Design review of the part built by this model. Coordinates are the model's own, in mm. A direction names the side the tool comes from. Give positions to 0.01 mm unless a question says otherwise; leave off trailing zeros. Write each loop counter-clockwise with the first axis right and the second up, starting at its lowest first coordinate (ties: lowest second). Pieces come first, ordered by that corner, then holes. Notation, with made-up numbers: (-23, -32.5) - (-7, -32.5) arc R10 ccw to (-7, -16.5) - close; hole circle Ø7 at (58.5, 7.5). An arc over 180 degrees is marked (long way). Use a Markdown table: item, result. Add a question column.
```python
from build123d import *

# Parameters (mm, degrees)
SKETCH1_R           = 5
BOSS_EXTRUDE1_DEPTH = 2
SKETCH2_R           = 3.9
BOSS_EXTRUDE2_DEPTH = 48
SKETCH3_R           = 2.5
BOSS_EXTRUDE3_DEPTH = 8


with BuildPart() as part:
    # Sketch1 → Boss-Extrude1 (new body)
    with BuildSketch(Plane(origin=(0, 0, 0), x_dir=(1, 0, 0), z_dir=(0, 1, 0))):
        Circle(SKETCH1_R)
    extrude(amount=BOSS_EXTRUDE1_DEPTH)

    # Sketch2 → Boss-Extrude2 (add)
    with BuildSketch(Plane(origin=(0, 2, 0), x_dir=(1, 0, 0), z_dir=(0, 1, 0))):
        Circle(SKETCH2_R)
    extrude(amount=BOSS_EXTRUDE2_DEPTH)

    # Sketch3 → Boss-Extrude3 (add)
    with BuildSketch(Plane(origin=(0, 50, 0), x_dir=(1, 0, 0), z_dir=(0, 1, 0))):
        Circle(SKETCH3_R)
    extrude(amount=BOSS_EXTRUDE3_DEPTH)


solid = part.part
```
(1) Add section D-D (z = -3.25). State the section outline as (x, y) points, and give its area (3 significant figures).
(2) Add section A-A (x = 0). State the section outline as (y, z) points, and give its area (3 significant figures).
(3) Tool access review of faces 1 (the face through (-0.54, 53.94, 2.44)), 2 (the face through (-1.08, 0.99, 4.88)): name each direction out of +Z, -Z, +X, -X, +Y, -Y from which nothing blocks a thin tool from reaching the whole face with its end or side.
(4) Insertion check: pin 1 (6 mm diameter, centred on y = 17.5, z = -2.5, fed in from -X); pin 2 (1 mm diameter, centred on y = 33.5, z = 1.5, fed in from -X); pin 3 (6 mm diameter, centred on x = -2.5, y = 34.5, fed in from -Z). Each pin has a flat end and moves straight along its axis. Give the tip position at first contact, or say it passes through.
(5) Add section B-B (z = 0). State the section outline as (x, y) points, and give its area (3 significant figures).
(6) For line 1 along Z through (x, y) = (0, 48); line 2 along Y through (x, z) = (-3.5, -0.25); line 3 along Y through (x, z) = (3.75, -3), list the stretches that pass through material, from the lowest coordinate up.
(7) Add section C-C (y = 26). State the section outline as (x, z) points.
Answers follow:
| question | item | result |
|---|---|---|
| 1 | outline | (-3.8, 0) - (3.8, 0) - (3.8, 2) - (2.16, 2) - (2.16, 50) - (-2.16, 50) - (-2.16, 2) - (-3.8, 2) - close |
| 1 | area | 222 mm^2 |
| 2 | outline | (0, -5) - (2, -5) - (2, -3.9) - (50, -3.9) - (50, -2.5) - (58, -2.5) - (58, 2.5) - (50, 2.5) - (50, 3.9) - (2, 3.9) - (2, 5) - (0, 5) - close |
| 2 | area | 434 mm^2 |
| 3 | face 1 | +Y |
| 3 | face 2 | +Y, -Y |
| 4 | pin 1 | x = -3.9 |
| 4 | pin 2 | x = -3.77 |
| 4 | pin 3 | z = -3.9 |
| 5 | outline | (-5, 0) - (5, 0) - (5, 2) - (3.9, 2) - (3.9, 50) - (2.5, 50) - (2.5, 58) - (-2.5, 58) - (-2.5, 50) - (-3.9, 50) - (-3.9, 2) - (-5, 2) - close |
| 5 | area | 434 mm^2 |
| 6 | line 1 | -3.9 to 3.9 |
| 6 | line 2 | 0 to 50 |
| 6 | line 3 | 0 to 2 |
| 7 | outline | circle Ø7.8 at (0, 0) |
